Input: part model. Units: mm. Frame: model coordinates. Face numbers are marked on the shaded views. A direction names the side the tool comes from. Round coordinates to 2 decimals unless told otherwise and drop trailing zeros. Order: outer loops, then holes, each group sorted by start corner. A loop starts at its lowest first (then second) coordinate and runs counter-clockwise, first axis right, second up. Notation, with made-up numbers: M -36,19 L -28,19 A23 ccw -28,37 Z; hole C 6.25,-36 d1. An arc over 180 degrees is marked long. One line per question, with ' | ' between items.
```python
from build123d import *

# Parameters (mm, degrees)
SKETCH1_R           = 30
BOSS_EXTRUDE1_DEPTH = 27.5
SKETCH3_R           = 5
CUT_EXTRUDE1_DEPTH  = 30
SKETCH5_R           = 4
BOSS_EXTRUDE2_DEPTH = 20


with BuildPart() as part:
    # Sketch1 → Boss-Extrude1 (new, symmetric)
    with BuildSketch(Plane.XY):
        Circle(SKETCH1_R)
    extrude(amount=BOSS_EXTRUDE1_DEPTH, both=True)

    # Sketch2 → Revolve2 (revolve)
    with BuildSketch(Plane.XY):
        Polygon((56.53339143, 45.869114373), (60.629151652, 43.001232191), (28.508871216, -2.871282289), (24.413110995, -0.003400107), align=None)
    revolve(axis=Axis((0, 0, 0), (0.5735764363510413, 0.8191520442889952, 0)))

    # Sketch3 → Cut-Extrude1 (cut, symmetric)
    with BuildSketch(Plane.XY):
        with Locations((31.546703999, 45.053362436)):
            Circle(SKETCH3_R)
    extrude(amount=CUT_EXTRUDE1_DEPTH, both=True, mode=Mode.SUBTRACT)

    # Sketch5 → Boss-Extrude2 (add)
    with BuildSketch(Plane.XY.offset(27.5)):
        Circle(SKETCH5_R)
    extrude(amount=BOSS_EXTRUDE2_DEPTH)


solid = part.part
```
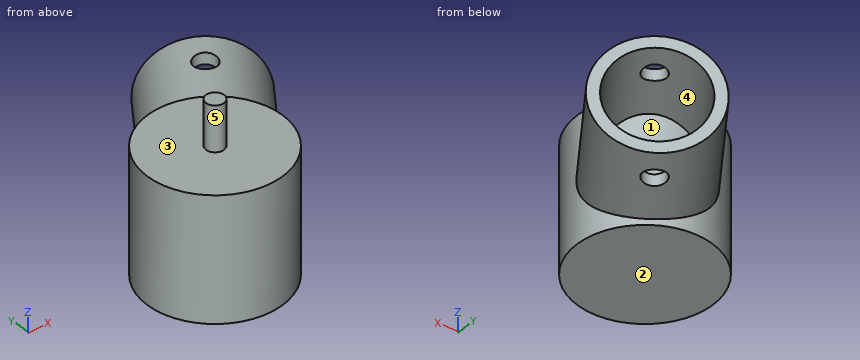
Item 1: Line query: line 1 along Z through (x, y) = (30, 38); line 2 along Z through (x, y) = (-16, 4.5); line 3 along Y through (x, z) = (7, -12.5). Output: solid intervals per line, ascending. Write a range as from..to.
Report:
line 1: -24.85..-19.81, 19.81..24.85 | line 2: -27.5..27.5 | line 3: -29.17..29.17, 37.22..47.74
Item 2: Section query B-B, the plane z = 29. Return loops of the section in (x, y).
Report:
outline: C 0,0 d8
Item 3: Mould query, pull axis Y, two halves, no side actions, for the marked faces 3, 4 and 5. Classes: +Y half, -Y half, draft (parallel to the pull), parting line (faces both ways), or undercut.
Report:
face 3: draft | face 4: undercut | face 5: parting line
Item 4: Access query for the marked faces 1 and 2. Directions: +Z, -Z, +X, -X, +Y, -Y. A direction counts if a zero-diameter tool reaches every point of the face in a straight line with its end or side. Return the directions, or none.
Report:
face 1: none | face 2: -Z, +X, -X, +Y, -Y
Item 5: Section query A-A, the plane z = -22.5. Return loops of the section in (x, y), plus the area to 3 significant figures.
Report:
outline: M 7.11,29.15 A30 ccw long 24.96,16.65 L 49.08,51.09 L 31.22,63.59 Z; hole C 31.55,45.05 d10 | area: 3,640 mm²
Item 6: Section query D-D, the plane y = -12. Return loops of the section in (x, z), plus the area to 3 significant figures.
Report:
outline: M -27.5,-27.5 L 27.5,-27.5 L 27.5,27.5 L -27.5,27.5 Z | area: 3,020 mm²
Item 7: Section query C-C, the plane x = -15.5. Return loops of the section in (y, z).
Report:
outline: M -25.69,-27.5 L 25.69,-27.5 L 25.69,27.5 L -25.69,27.5 Z
Item 8: First-contact query: pin 1 (1.5 mm diameter, centred on x = -10.5, y = 21, fed in from +Z); pin 2 (11.5 mm diameter, centred on x = 31.55, y = 45.05, fed in from -Z); pin 3 (3 mm diameter, centred on y = 18.5, z = -9.5, fed in from +X); pin 4 (8 mm diameter, centred on x = 31.55, y = 45.05, fed in from -Z). Flat tips, straight axial feed; report the tip coordinate or a pass-through.
Report:
pin 1: z = 27.5 | pin 2: z = -25 | pin 3: x = 42.45 | pin 4: through
